Autodesk Inventor part; units mm, degrees
ref_plane "YZ Plane" through (0, 0, 0) normal (1, 0, 0) x (0, 1, 0)
ref_plane "XZ Plane" through (0, 0, 0) normal (0, 1, 0) x (-1, 0, 0)
ref_plane "XY Plane" through (0, 0, 0) normal (0, 0, 1) x (1, 0, 0)
sketch "Sketch1" plane through (0, 0, 0) normal (0, 0, 1) x (1, 0, 0)
  line L0 (0, 0) -> (127, 0)
  line L1 (127, 0) -> (127, 76.2)
  line L2 (127, 76.2) -> (0, 76.2)
  line L3 (0, 76.2) -> (0, 0)
  dimension "d0" = 127
  dimension "d1" = 76.2
extrude "Extrusion1" add sketch "Sketch1" along normal blind 9.525
sketch "Sketch2" plane through (0, 0, 9.525) normal (0, 0, 1) x (1, 0, 0)
  line L0 (127, 0) -> (0, 0)
  line L1 (0, 76.2) -> (127, 76.2)
  line L2 (44.45, 0) -> (82.55, 0)
  line L3 (82.55, 0) -> (82.55, 6.35)
  line L4 (82.55, 6.35) -> (44.45, 6.35)
  line L5 (44.45, 6.35) -> (44.45, 0)
  line L6 (63.5, 76.2) -> (63.5, 0) construction
  dimension "d4" = 38.1
  dimension "d5" = 6.35
extrude "Extrusion2" add sketch "Sketch2" along normal blind 9.525
ref_plane "Work Plane1" through (0, 38.1, 0) normal (0, 1, 0) x (1, 0, 0)
ref_plane "Work Plane2" through (63.5, 0, 0) normal (1, 0, 0) x (0, 0, -1)
sketch "Sketch3" plane through (0, 0, 9.525) normal (0, 0, 1) x (1, 0, 0)
  line L0 (0, 0) -> (0, 76.2)
  line L1 (127, 76.2) -> (127, 0)
  line L2 (127, 53.975) -> (120.65, 53.975)
  line L3 (120.65, 53.975) -> (120.65, 22.225)
  line L4 (120.65, 22.225) -> (127, 22.225)
  line L5 (127, 22.225) -> (127, 53.975)
  line L6 (0, 38.1) -> (127, 38.1) construction
  point P0 (63.5, 38.1)
  dimension "d8" = 31.75
  dimension "d9" = 6.35
extrude "Extrusion3" add sketch "Sketch3" along normal blind 9.525
sketch "Sketch4" plane through (0, 0, 19.05) normal (0, 0, 1) x (1, 0, 0)
  line L0 (44.45, 0) -> (82.55, 0)
  line L1 (82.55, 0) -> (82.55, 12.7)
  line L2 (82.55, 12.7) -> (44.45, 12.7)
  line L3 (44.45, 12.7) -> (44.45, 0)
  point P0 (44.45, 6.35)
  point P1 (82.55, 6.35)
  point P2 (0, 0)
  dimension "d12" = 38.1
  dimension "d13" = 38.1
  dimension "d14" = 12.7
extrude "Extrusion4" add sketch "Sketch4" along normal blind 6.35
sketch "Sketch5" plane through (0, 0, 19.05) normal (0, 0, 1) x (1, 0, 0)
  line L0 (127, 53.975) -> (114.3, 53.975)
  line L1 (114.3, 53.975) -> (114.3, 22.225)
  line L2 (114.3, 22.225) -> (127, 22.225)
  line L3 (127, 22.225) -> (127, 53.975)
  point P0 (0, 0)
  dimension "d17" = 31.75
  dimension "d18" = 31.75
  dimension "d19" = 12.7
extrude "Extrusion5" add sketch "Sketch5" along normal blind 6.35
mirror "Mirror3" about plane through (0, 38.1, 0) normal (0, 1, 0) of "Extrusion2", "Extrusion4"
mirror "Mirror4" about plane through (63.5, 0, 0) normal (1, 0, 0) of "Extrusion3", "Extrusion5"
ref_plane "Work Plane3" through (0, 0, 4.7625) normal (0, 0, 1) x (1, 0, 0)
mirror "Mirror5" about plane through (0, 0, 4.7625) normal (0, 0, 1) of "Extrusion2", "Extrusion4", "Mirror3", "Extrusion3", "Extrusion5", "Mirror4"
equation "\"d12\" = d13"
equation "\"d18\" = d17"
properties part number "Rover Electronics Raft"
Model file for the job. Use its own axes, mm. A direction names the side the tool comes from. Give positions to 0.01 mm unless a question says otherwise; leave off trailing zeros. Write each loop counter-clockwise with the first axis right and the second up, starting at its lowest first coordinate (ties: lowest second). Pieces come first, ordered by that corner, then holes. Notation, with made-up numbers: M 81,14 L 116,14 A14 ccw 116,22 Z; hole C 79.25,0.5 d10. An arc over 180 degrees is marked long. One line per item, written item: value. Start each with the question number.
Q1. Saw through at D-D, the plane y = 36. Write the cut outline in (x, z) (3 decimals).
Q2. Saw through at C-C, the plane x = 55.5. Write the cut outline in (y, z) (3 decimals).
Q3. Probe probe 1 along X at (y, z) = (45, 22); probe 2 along Y at (x, z) = (49, -1.5); probe 3 along X at (y, z) = (46.5, -7.5). List the from-to ranges inside material, lowest first. Write a range as [from, to].
Q4. Drop flat-ended pins along their axis: pin 1 Ø4 at (x, z) = (121.5, 16) entering from -Y (3 decimals); pin 2 Ø6.5 at (y, z) = (7, 17.5) entering from +X; pin 3 Ø6.5 at (x, z) = (6.5, 20) entering from +Y (3 decimals). Give the stop position or say it passes through.
Q5. Saw through at A-A, the plane y = 67.5. Write the cut outline in (x, z) (3 decimals), plus the area to 3 significant figures.
Q6. 3-axis set-ups, long thin cutter, end or side, ignore diameter. For faces 4 (the flat face through (82.55, 71, -10)), 5 (the flat face through (63, 63.5, 22)), 6 (the flat face through (63, 6.35, -5)), 7 (the flat face through (82.55, 5, 19)), 8 (the flat face through (122, 53.975, -10)): which of +Z, -Z, +X, -X, +Y, -Y reach the whole face in a straight line?
Q7. Saw through at B-B, the plane z = -5. Write the cut outline in (x, y) (3 decimals).
Q8. Two-plate mould, pull along Z, no slides. Class faces 1 (the flat face through (114.3, 38, -13)), 2 (the flat face through (6, 38, 25.4)), 3 (the flat face through (63, 69.85, 14)): +Z half, -Z half, draft (parallel to the pull), parting line (faces both ways), or undercut.
Output values:
1. outline: M 0,-15.875 L 12.7,-15.875 L 12.7,-9.525 L 6.35,-9.525 L 6.35,0 L 120.65,0 L 120.65,-9.525 L 114.3,-9.525 L 114.3,-15.875 L 127,-15.875 L 127,25.4 L 114.3,25.4 L 114.3,19.05 L 120.65,19.05 L 120.65,9.525 L 6.35,9.525 L 6.35,19.05 L 12.7,19.05 L 12.7,25.4 L 0,25.4 Z
2. outline: M 0,-15.875 L 12.7,-15.875 L 12.7,-9.525 L 6.35,-9.525 L 6.35,0 L 69.85,0 L 69.85,-9.525 L 63.5,-9.525 L 63.5,-15.875 L 76.2,-15.875 L 76.2,25.4 L 63.5,25.4 L 63.5,19.05 L 69.85,19.05 L 69.85,9.525 L 6.35,9.525 L 6.35,19.05 L 12.7,19.05 L 12.7,25.4 L 0,25.4 Z
3. probe 1: x = [0, 12.7], [114.3, 127]
3. probe 2: y = [0, 6.35], [69.85, 76.2]
3. probe 3: x = [0, 6.35], [120.65, 127]
4. pin 1: stops at y = 22.225
4. pin 2: stops at x = 82.55
4. pin 3: stops at y = 53.975
5. outline: M 0,0 L 127,0 L 127,9.525 L 0,9.525 Z; M 44.45,-15.875 L 82.55,-15.875 L 82.55,-9.525 L 44.45,-9.525 Z; M 44.45,19.05 L 82.55,19.05 L 82.55,25.4 L 44.45,25.4 Z
5. area: 1,690 mm²
6. face 4: -Z, +X, +Y, -Y
6. face 5: +Z, +X, -X
6. face 6: +X, -X
6. face 7: +Z, +X, +Y, -Y
6. face 8: -Z, +X, -X, +Y
7. outline: M 0,22.225 L 6.35,22.225 L 6.35,53.975 L 0,53.975 Z; M 44.45,0 L 82.55,0 L 82.55,6.35 L 44.45,6.35 Z; M 44.45,69.85 L 82.55,69.85 L 82.55,76.2 L 44.45,76.2 Z; M 120.65,22.225 L 127,22.225 L 127,53.975 L 120.65,53.975 Z
8. face 1: draft
8. face 2: +Z half
8. face 3: undercut
